Geometry check sheet. Reference: drawing and pictorial views, mm from the part's lowest x, y, z. A direction names the side the tool comes from. Coordinates: 2 decimals unless noted, no trailing zeros. Loops run counter-clockwise (first coordinate to the right, second up) from the corner with the lowest first, then second, coordinate; pieces in that order, holes last. Notation, with made-up numbers: (-1.75, 85) -> (27.25, 85) arc R16 ccw to (27.25, 111) -> close; hole circle Ø3 at (40.5, 0). An arc over 180 degrees is marked (long way). Answer as a JSON object with one key per item and string values.
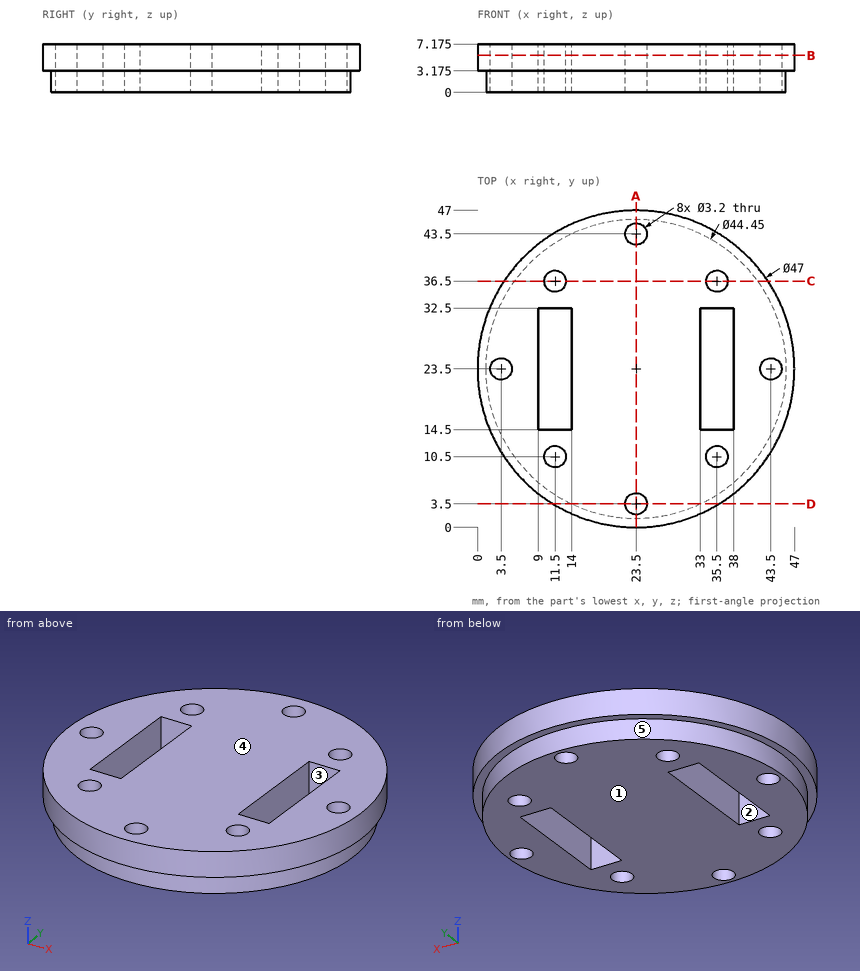
1. Section check C-C, the plane y = 36.5. Record the boundary of the cut face in (x, z) (3 decimals), then the cut area to 3 significant figures.
Evaluation:
{"outline": "(3.923, 3.175) -> (5.474, 3.175) -> (5.474, 0) -> (9.9, 0) -> (9.9, 7.175) -> (3.923, 7.175) -> close; (13.1, 0) -> (33.9, 0) -> (33.9, 7.175) -> (13.1, 7.175) -> close; (37.1, 0) -> (41.526, 0) -> (41.526, 3.175) -> (43.077, 3.175) -> (43.077, 7.175) -> (37.1, 7.175) -> close", "area": "225 mm^2"}
2. Tool access check on the marked faces 1 and 2. Record the directions out of +Z, -Z, +X, -X, +Y, -Y that give a thin tool (end or side, any length) a straight path to the whole face; none if there is none.
Evaluation:
{"face 1": "-Z, +X, -X, +Y, -Y", "face 2": "+Z, -Z"}
3. Mould release check, pull along Y, two halves, no side actions. Record for the marked faces 3, 4 and 5: released by +Y, released by -Y, zero draft, split by the parting line, or undercut.
Evaluation:
{"face 3": "undercut", "face 4": "zero draft", "face 5": "split by the parting line"}
4. Section check B-B, the plane z = 5.5. State how many separate pieces and enclosed holes the cut face has, then the cut area to 3 significant figures.
Evaluation:
{"separate pieces": "1", "enclosed holes": "10", "area": "1,490 mm^2"}
5. Depth check by flat-ended pin: P1, Ø4, axis at x = 10.5, z = 5, coming from the +Y side; P2, Ø3, axis at x = 39, z = 2.5, coming from the +Y side; P3, Ø3.5, axis at y = 21, z = 3.5, coming from the +X side. Enter the tip coordinate at first touch or a pass-through.
Evaluation:
{"P1": "stops at y = 44.27", "P2": "stops at y = 42.25", "P3": "stops at x = 46.99"}
6. Section check A-A, the plane x = 23.5. Record the boundary of the cut face in (y, z) (3 decimals).
Evaluation:
{"outline": "(0, 3.175) -> (1.275, 3.175) -> (1.275, 0) -> (1.9, 0) -> (1.9, 7.175) -> (0, 7.175) -> close; (5.1, 0) -> (41.9, 0) -> (41.9, 7.175) -> (5.1, 7.175) -> close; (45.1, 0) -> (45.725, 0) -> (45.725, 3.175) -> (47, 3.175) -> (47, 7.175) -> (45.1, 7.175) -> close"}
7. Thickness scan on probe 1 along Y at (x, z) = (23.5, 5.5); probe 2 along X at (y, z) = (19.5, 4); probe 3 along Y at (x, z) = (11.5, 2.75). Record the ranges inside material, lowest first. Write a range as from..to.
Evaluation:
{"probe 1": "y = 0..1.9, 5.1..41.9, 45.1..47", "probe 2": "x = 0.34..9, 14..33, 38..46.66", "probe 3": "y = 4.79..8.9, 12.1..14.5, 32.5..34.9, 38.1..42.21"}
8. Section check D-D, the plane y = 3.5. Record the boundary of the cut face in (x, z) (3 decimals).
Evaluation:
{"outline": "(11.161, 3.175) -> (13.807, 3.175) -> (13.807, 0) -> (21.9, 0) -> (21.9, 7.175) -> (11.161, 7.175) -> close; (25.1, 0) -> (33.193, 0) -> (33.193, 3.175) -> (35.839, 3.175) -> (35.839, 7.175) -> (25.1, 7.175) -> close"}
